Geometry check sheet. Reference: drawing and pictorial views, mm from the part's lowest x, y, z. A direction names the side the tool comes from. Give positions to 0.01 mm unless a question says otherwise; leave off trailing zeros. Order: outer loops, then holes, each group sorted by start corner. A loop starts at its lowest first (then second) coordinate and runs counter-clockwise, first axis right, second up.
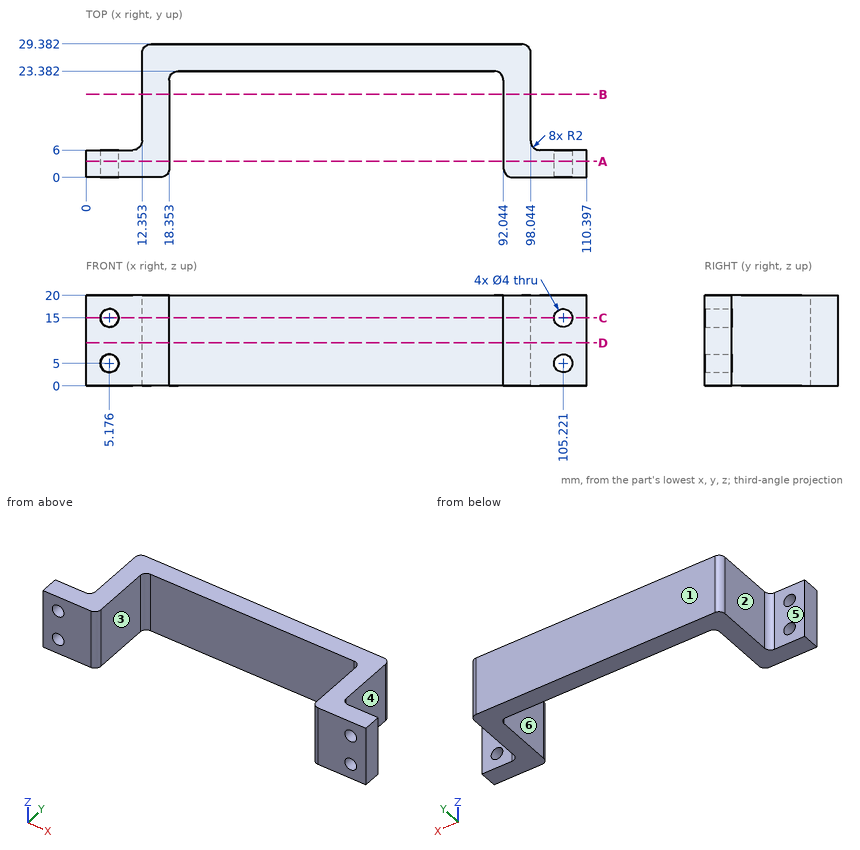
(1) Gauge pin test, flat ends, axial feed: pin 1 Ø9.5 at (y, z) = (17, 7.5) entering from -X; pin 2 Ø6 at (y, z) = (16.5, 5) entering from +X (1 decimal); pin 3 Ø2 at (x, z) = (53.5, 5.5) entering from -Y. Record the tip position at first contact, or that the pin passes through.
Response values:
pin 1: stops at x = 12.35
pin 2: stops at x = 98
pin 3: stops at y = 23.38
(2) Cross-section at D-D on z = 9.5. Enter the section's corners in (x, y) (1 decimal).
Response values:
outline: (0, 0) - (16.4, 0) arc R2 ccw to (18.4, 2) - (18.4, 21.4) arc R2 cw to (20.4, 23.4) - (90, 23.4) arc R2 cw to (92, 21.4) - (92, 2) arc R2 ccw to (94, 0) - (110.4, 0) - (110.4, 6) - (100, 6) arc R2 cw to (98, 8) - (98, 27.4) arc R2 ccw to (96, 29.4) - (14.4, 29.4) arc R2 ccw to (12.4, 27.4) - (12.4, 8) arc R2 cw to (10.4, 6) - (0, 6) - close
(3) Cross-section at A-A on y = 3.5. Enter the section's corners in (x, z) (1 decimal).
Response values:
outline: (0, 0) - (18.4, 0) - (18.4, 20) - (0, 20) - close; (92, 0) - (110.4, 0) - (110.4, 20) - (92, 20) - close; hole circle Ø4 at (5.2, 5); hole circle Ø4 at (5.2, 15); hole circle Ø4 at (105.2, 5); hole circle Ø4 at (105.2, 15)
(4) Set-up check for the marked faces 1, 2 and 3: record each of +Z, -Z, +X, -X, +Y, -Y from which the full face is reachable in a straight line by a thin tool's end or side.
Response values:
face 1: +Z, -Z, +X, -X, +Y
face 2: +Z, -Z, -X, +Y
face 3: +Z, -Z, -Y
(5) Release check for a two-part mould opening along X. For the marked faces 4, 5 and 6 record: released by +X, released by -X, zero draft, split by the parting line, or undercut.
Response values:
face 4: released by +X
face 5: zero draft
face 6: undercut
(6) Cross-section at B-B on y = 18.25. Enter the section's corners in (x, z) (1 decimal), then the cut area to 3 significant figures.
Response values:
outline: (12.4, 0) - (18.4, 0) - (18.4, 20) - (12.4, 20) - close; (92, 0) - (98, 0) - (98, 20) - (92, 20) - close
area: 240 mm2
(7) Cross-section at C-C on z = 15. Enter the section's corners in (x, y) (1 decimal).
Response values:
outline: (0, 0) - (3.2, 0) - (3.2, 6) - (0, 6) - close; (7.2, 0) - (16.4, 0) arc R2 ccw to (18.4, 2) - (18.4, 21.4) arc R2 cw to (20.4, 23.4) - (90, 23.4) arc R2 cw to (92, 21.4) - (92, 2) arc R2 ccw to (94, 0) - (103.2, 0) - (103.2, 6) - (100, 6) arc R2 cw to (98, 8) - (98, 27.4) arc R2 ccw to (96, 29.4) - (14.4, 29.4) arc R2 ccw to (12.4, 27.4) - (12.4, 8) arc R2 cw to (10.4, 6) - (7.2, 6) - close; (107.2, 0) - (110.4, 0) - (110.4, 6) - (107.2, 6) - close
(8) Material ranges on L1, parallel to X at y = 3.9, z = 15 (1 decimal); L2, parallel to X at y = 18, z = 7.5 (1 decimal); L3, parallel to Y at x = 21.5, z = 9.5, recorded low to high.
Response values:
L1: x = 0 to 3.2, 7.2 to 18.4, 92 to 103.2, 107.2 to 110.4
L2: x = 12.4 to 18.4, 92 to 98
L3: y = 23.38 to 29.38
